Can you work these out from the drawing? Everything is in mm from the part's minimum corner. Give positions to 0.01 mm unless a question says otherwise; leave off trailing zeros. Write each loop counter-clockwise with the first axis right and the second up, starting at its lowest first coordinate (ties: lowest second). Pieces come first, ordered by that corner, then holes. Notation, with made-up numbers: (85.5, 60.25) - (128.5, 60.25) arc R19 ccw to (128.5, 87.25) - close; hole circle Ø5 at (25.5, 49.5). An arc over 180 degrees is marked (long way). Write each question's results on one line, items separated by ' | '. Start each with the question number.
Item 1: Suppose I cut it at C-C on x = 6. List the corners of the cut face in (y, z) for me, then the cut area to 3 significant figures.
Item 2: Suppose I cut it at B-B on x = 161. List the corners of the cut face in (y, z) for me, then the cut area to 3 significant figures.
Item 3: Suppose I cut it at D-D on z = 81. List the corners of the cut face in (x, y) for me, then the cut area to 3 significant figures.
Item 4: Will these pins go through, and if not, where does the flat tip stop? P1, Ø3.5, axis at x = 161, z = 15, coming from the -Y side; P2, Ø6.5, axis at x = 6, z = 30, coming from the -Y side.
Item 5: Please list where these lines run through material, in increasing order: line 1 along Z through (x, y) = (6, 5.2); line 2 along Z through (x, y) = (6, 2.8); line 3 along Z through (x, y) = (161, 1.9).
Item 6: Suppose I cut it at A-A on z = 15. List the corners of the cut face in (x, y) for me, then the cut area to 3 significant figures.
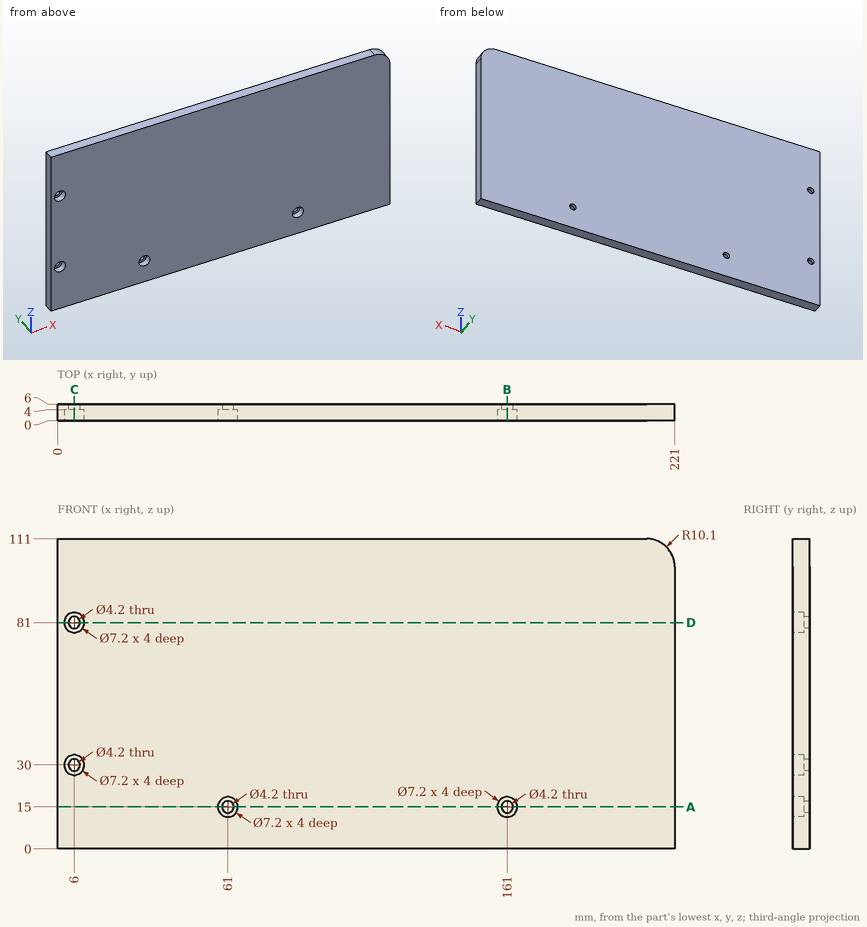
Checked values:
1) outline: (0, 0) - (6, 0) - (6, 27.9) - (4, 27.9) - (4, 26.4) - (0, 26.4) - close; (0, 33.6) - (4, 33.6) - (4, 32.1) - (6, 32.1) - (6, 78.9) - (4, 78.9) - (4, 77.4) - (0, 77.4) - close; (0, 84.6) - (4, 84.6) - (4, 83.1) - (6, 83.1) - (6, 111) - (0, 111) - close | area: 592 mm^2
2) outline: (0, 0) - (6, 0) - (6, 12.9) - (4, 12.9) - (4, 11.4) - (0, 11.4) - close; (0, 18.6) - (4, 18.6) - (4, 17.1) - (6, 17.1) - (6, 111) - (0, 111) - close | area: 629 mm^2
3) outline: (0, 0) - (2.4, 0) - (2.4, 4) - (3.9, 4) - (3.9, 6) - (0, 6) - close; (8.1, 4) - (9.6, 4) - (9.6, 0) - (221, 0) - (221, 6) - (8.1, 6) - close | area: 1,290 mm^2
4) P1: passes through | P2: stops at y = 4
5) line 1: z = 0 to 27.9, 32.1 to 78.9, 83.1 to 111 | line 2: z = 0 to 26.4, 33.6 to 77.4, 84.6 to 111 | line 3: z = 0 to 11.4, 18.6 to 111
6) outline: (0, 0) - (57.4, 0) - (57.4, 4) - (58.9, 4) - (58.9, 6) - (0, 6) - close; (63.1, 4) - (64.6, 4) - (64.6, 0) - (157.4, 0) - (157.4, 4) - (158.9, 4) - (158.9, 6) - (63.1, 6) - close; (163.1, 4) - (164.6, 4) - (164.6, 0) - (221, 0) - (221, 6) - (163.1, 6) - close | area: 1,250 mm^2
